from build123d import *

# Parameters (mm, degrees)
SKETCH1_W                       = 127
SKETCH1_H                       = 114.3
STOCK_DEPTH                     = 9.525
NUC_STANDOFFS_D                 = 2.2606
COVER_MOUNT_D                   = 2.2606
FILLET1_R                       = 3.175
LIDAR_BOX_MOUNT_D               = 2.2606
F_1_4_20_TAPPED_HOLE1_D         = 5.1054
F_21_0_159_DIAMETER_HOLE1_D     = 4.0386
F_21_0_159_DIAMETER_HOLE1_DEPTH = 9.525
O_0_316_DIAMETER_HOLE1_D        = 8.0264
O_0_316_DIAMETER_HOLE1_DEPTH    = 9.525


with BuildPart() as part:
    # Sketch1 → stock (new body)
    with BuildSketch(Plane(origin=(0, 0, 0), x_dir=(1, 0, 0), z_dir=(0, 1, 0))):
        Rectangle(SKETCH1_W, SKETCH1_H)
    extrude(amount=STOCK_DEPTH)

    # NUC standoffs (through all)
    with Locations(Plane(origin=(0, 9.525, 0), x_dir=(1, 0, 0), z_dir=(0, 1, 0))):
        with Locations((-47.499999996, 45.200000024), (-47.499999996, -45.200000024), (47.499999996, -45.200000024), (47.499999996, 45.200000024), (0, 0)):
            Hole(NUC_STANDOFFS_D / 2)

    # Cover mount (through all)
    with Locations(Plane(origin=(0, 9.525, 0), x_dir=(1, 0, 0), z_dir=(0, 1, 0))):
        with Locations((60.325, 25.4), (60.325, -25.4), (-60.325, -25.4), (-60.325, 25.4), (0, 0)):
            Hole(COVER_MOUNT_D / 2)

    # Fillet1
    fillet1_edges = [part.edges().sort_by_distance(p)[0] for p in [
        (-63.5, 4.7625, -57.15),
        (63.5, 4.7625, -57.15),
        (63.5, 4.7625, 57.15),
        (-63.5, 4.7625, 57.15),
    ]]
    fillet(fillet1_edges, radius=FILLET1_R)

    # lidar box mount (through all)
    with Locations(Plane(origin=(0, 9.525, 0), x_dir=(1, 0, 0), z_dir=(0, 1, 0))):
        with Locations((0, -47.625), (0, 47.625)):
            Hole(LIDAR_BOX_MOUNT_D / 2)

    # 1/4-20 Tapped Hole1 (through all)
    with Locations(Plane(origin=(50.8, 0, -38.1), x_dir=(0, 0, -1), z_dir=(0, -1, 0))):
        with Locations((0, 0), (0, -25.4), (-38.1, -25.4), (-38.1, 0), (-76.2, 0), (-76.2, -25.4), (-76.2, -76.2), (-76.2, -101.6), (-38.1, -101.6), (-38.1, -76.2), (0, -76.2), (0, -101.6)):
            Hole(F_1_4_20_TAPPED_HOLE1_D / 2)

    # #21 (0.159) Diameter Hole1
    with Locations(Plane(origin=(0, 0, 0), x_dir=(-1, 0, 0), z_dir=(0, -1, 0))):
        with Locations((-47.499999996, 45.200000024), (-60.325, 25.4), (-60.325, -25.4), (-47.499999996, -44.069700024), (0, -47.625), (47.499999996, -45.200000024), (60.325, -25.4), (60.325, 25.4), (47.499999996, 45.200000024), (0, 47.625)):
            Hole(F_21_0_159_DIAMETER_HOLE1_D / 2, depth=F_21_0_159_DIAMETER_HOLE1_DEPTH)

    # O (0.316) Diameter Hole1
    with Locations(Plane(origin=(0, 0, 0), x_dir=(-1, 0, 0), z_dir=(0, -1, 0))):
        with Locations((-50.8, 38.1), (-25.4, 38.1), (-25.4, 0), (-50.8, 0), (-50.8, -38.1), (-25.4, -38.1), (25.4, -38.1), (50.8, -38.1), (50.8, 0), (25.4, 0), (25.4, 38.1), (50.8, 38.1)):
            Hole(O_0_316_DIAMETER_HOLE1_D / 2, depth=O_0_316_DIAMETER_HOLE1_DEPTH)


solid = part.part
The listing builds one solid part. Answer for the finished solid, in the listing's coordinates (mm). Round coordinates to 2 decimals unless told otherwise and drop trailing zeros. Write each loop counter-clockwise with the first axis right and the second up, starting at its lowest first coordinate (ties: lowest second). Pieces come first, ordered by that corner, then holes. Notation, with made-up numbers: (77.25, -19.5) - (134.25, -19.5) arc R9 cw to (134.25, -8.5) - close; hole circle Ø8 at (74.25, -31). An arc over 180 degrees is marked (long way). Use one line per item in the form item = value. Start each with the question number.
Item 1: A cutting plane is placed at D-D (y = 7.25). Give the number of separate pieces and of enclosed holes in the cut face, plus the area to 3 significant figures.
Item 2: A cutting plane is placed at B-B (z = 38.1). Write down the section's boundary in (x, y) (3 decimals).
Item 3: A cutting plane is placed at A-A (x = -25.4). Write down the section's boundary in (y, z) (3 decimals), plus the area to 3 significant figures.
Item 4: A cutting plane is placed at C-C (z = 25.4). Write down the section's boundary in (x, y) (3 decimals), plus the area to 3 significant figures.
Item 5: A flat-ended cylindrical pin translates along its axis: pin 1 Ø7 at (x, z) = (-50.8, 0) entering from +Y. Find the tip coordinate at first contact, or state that the pin passes through.
Item 6: Find the intervals of material crossed by line 1 (X direction, y = 6.5, z = -38.1); line 2 (X direction, y = 6.75, z = -25.4); line 3 (Z direction, x = 0, y = 3.25), in increasing order. Write a range as [from, to].
Item 7: Determine the mould class of faces 1 (the cylindrical face through (-47.94, 4.83, 47.17)), 2 (the flat face through (63.5, 5, 1)), 3 (the flat face through (-1, 5, 57.15)) for opening direction X: +X half, -X half, draft (parallel to the pull), parting line (faces both ways), or undercut.
The answers:
q1.separate_pieces = 1
q1.enclosed_holes = 23
q1.area = 13,800 mm^2
q2.outline = (-63.5, 0) - (-54.813, 0) - (-54.813, 9.525) - (-63.5, 9.525) - close; (-46.787, 0) - (-29.413, 0) - (-29.413, 9.525) - (-46.787, 9.525) - close; (-21.387, 0) - (21.387, 0) - (21.387, 9.525) - (-21.387, 9.525) - close; (29.413, 0) - (46.787, 0) - (46.787, 9.525) - (29.413, 9.525) - close; (54.813, 0) - (63.5, 0) - (63.5, 9.525) - (54.813, 9.525) - close
q3.outline = (0, -57.15) - (9.525, -57.15) - (9.525, -42.113) - (0, -42.113) - close; (0, -34.087) - (9.525, -34.087) - (9.525, -4.013) - (0, -4.013) - close; (0, 4.013) - (9.525, 4.013) - (9.525, 34.087) - (0, 34.087) - close; (0, 42.113) - (9.525, 42.113) - (9.525, 57.15) - (0, 57.15) - close
q3.area = 859 mm^2
q4.outline = (-63.5, 0) - (-62.344, 0) - (-62.344, 9.525) - (-63.5, 9.525) - close; (-58.306, 0) - (58.306, 0) - (58.306, 9.525) - (-58.306, 9.525) - close; (62.344, 0) - (63.5, 0) - (63.5, 9.525) - (62.344, 9.525) - close
q4.area = 1,130 mm^2
q5.pin_1 = through
q6.line_1 = [-63.5, -54.81], [-46.79, -29.41], [-21.39, 21.39], [29.41, 46.79], [54.81, 63.5]
q6.line_2 = [-63.5, -62.34], [-58.31, 58.31], [62.34, 63.5]
q6.line_3 = [-57.15, -49.64], [-45.61, -1.13], [1.13, 45.61], [49.64, 57.15]
q7.face_1 = undercut
q7.face_2 = +X half
q7.face_3 = draft
